For this review, use the dimensioned drawing (mm, ordinates from the lowest corner) and the shaded views. A direction names the side the tool comes from. Coordinates: 2 decimals unless noted, no trailing zeros. Order: outer loops, then holes, each group sorted by start corner. A loop starts at its lowest first (then second) coordinate and runs counter-clockwise, first axis right, second up. Notation, with made-up numbers: M 16,83 L 74,83 A9 cw 74,96 Z; hole C 79.25,16 d1. An arc over 180 degrees is marked long. One line per item, written item: value.
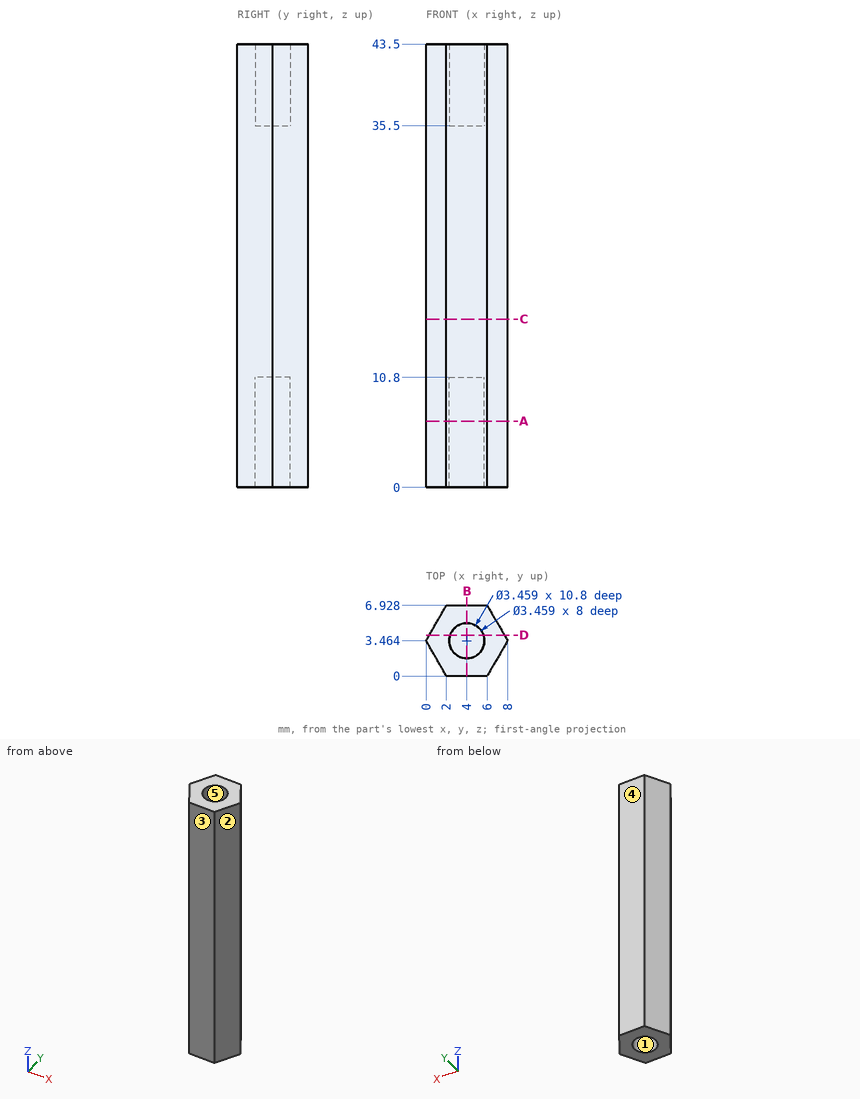
(1) Insertion check: pin 1 Ø1.7 at (x, y) = (4, 3) entering from -Z; pin 2 Ø4 at (y, z) = (1.5, 20) entering from +X; pin 3 Ø3 at (y, z) = (5.5, 19.5) entering from -X. Each pin has a flat end and moves straight along its axis. Give the tip position at first contact, or say it passes through.
Geometry results:
pin 1: stops at z = 10.8
pin 2: stops at x = 8
pin 3: stops at x = 0.31
(2) Mouldability with a two-part tool opening along Y and no side actions: class the marked faces 3, 4 and 5 as +Y half, -Y half, draft (parallel to the pull), parting line (faces both ways), or undercut.
Geometry results:
face 3: -Y half
face 4: +Y half
face 5: undercut
(3) We need section D-D, the plane y = 4. State the section outline as (x, z) points, plus the area to 3 significant figures.
Geometry results:
outline: M 0.31,0 L 2.36,0 L 2.36,10.8 L 5.64,10.8 L 5.64,0 L 7.69,0 L 7.69,43.5 L 5.64,43.5 L 5.64,35.5 L 2.36,35.5 L 2.36,43.5 L 0.31,43.5 Z
area: 259 mm2
(4) Tool access review of the marked faces 1 and 2: name each direction out of +Z, -Z, +X, -X, +Y, -Y from which nothing blocks a thin tool from reaching the whole face with its end or side.
Geometry results:
face 1: -Z
face 2: +Z, -Z, +X, -Y
(5) We need section B-B, the plane x = 4. State the section outline as (y, z) points (1 decimal), plus the area to 3 significant figures.
Geometry results:
outline: M 0,0 L 1.7,0 L 1.7,10.8 L 5.2,10.8 L 5.2,0 L 6.9,0 L 6.9,43.5 L 5.2,43.5 L 5.2,35.5 L 1.7,35.5 L 1.7,43.5 L 0,43.5 Z
area: 236 mm2
(6) For L1, parallel to X at y = 4.75, z = 9 (1 decimal); L2, parallel to Z at x = 4.5, y = 2; L3, parallel to Y at x = 3, z = 42 (1 decimal), list the stretches that pass through material, from the lowest coordinate up.
Geometry results:
L1: x = 0.7 to 2.8, 5.2 to 7.3
L2: z = 10.8 to 35.5
L3: y = 0 to 2.1, 4.9 to 6.9
(7) We need section A-A, the plane z = 6.5. State the section outline as (x, y) points.
Geometry results:
outline: M 0,3.46 L 2,0 L 6,0 L 8,3.46 L 6,6.93 L 2,6.93 Z; hole C 4,3.46 d3.46
(8) We need section C-C, the plane z = 16.5. State the section outline as (x, y) points.
Geometry results:
outline: M 0,3.46 L 2,0 L 6,0 L 8,3.46 L 6,6.93 L 2,6.93 Z
